```python
from build123d import *

# Parameters (mm, degrees)
SKETCH_1_R          = 8
SKETCH_1_R_2        = 6
EXTRUDE_1_DEPTH     = 2
SKETCH_1_3_R        = 6
SKETCH_1_3_R_2      = 1.65
EXTRUDE_2_DEPTH     = 35
SKETCH_2_R          = 1
CUT_EXTRUDE_1_DEPTH = 2
CUT_EXTRUDE_START   = 35
SKETCH_1_4_R        = 1.65
CUT_EXTRUDE_2_DEPTH = 13
CHAMFER_1_SIZE      = 0.2
CHAMFER_2_SIZE      = 0.3


with BuildPart() as part:
    # 스케치1 → 보스-돌출1 (new body)
    with BuildSketch(Plane(origin=(0, 0, 0), x_dir=(1, 0, 0), z_dir=(0, 1, 0))):
        with Locations(Location((0, 0, 0), (0, 0, 270))):
            Circle(SKETCH_1_R)
        with Locations(Location((0, 0, 0), (0, 0, 270))):
            Circle(SKETCH_1_R_2, mode=Mode.SUBTRACT)
    extrude(amount=EXTRUDE_1_DEPTH)

    # 스케치1<3> → 보스-돌출2 (add)
    # profile 1 of 2: a face of its own
    with BuildSketch(Plane(origin=(0, 0, 0), x_dir=(1, 0, 0), z_dir=(0, 1, 0))):
        with Locations(Location((0, 0, 0), (0, 0, 270))):
            Circle(SKETCH_1_3_R)
        Circle(SKETCH_1_3_R_2, mode=Mode.SUBTRACT)
    # profile 2 of 2: a face of its own
    with BuildSketch(Plane(origin=(0, 0, 0), x_dir=(1, 0, 0), z_dir=(0, 1, 0))):
        Circle(SKETCH_1_3_R_2)
    extrude(amount=EXTRUDE_2_DEPTH)

    # 스케치2 → 컷-돌출1 (cut)
    with BuildSketch(Plane.XZ):
        with Locations((0, 3)):
            Circle(SKETCH_2_R)
        with BuildLine():
            ThreePointArc((1, 3), (0, 2), (-1, 3))
            Line((-1, 3), (-1, -3))
            ThreePointArc((-1, -3), (0, -2), (1, -3))
            Line((1, -3), (1, 3))
        make_face()
        with Locations((0, -3)):
            Circle(SKETCH_2_R)
    extrude(amount=-CUT_EXTRUDE_1_DEPTH, mode=Mode.SUBTRACT)

    # 스케치1<4> → 컷-돌출2 (cut)
    with BuildSketch(Plane(origin=(0, 0, 0), x_dir=(1, 0, 0), z_dir=(0, 1, 0)).offset(CUT_EXTRUDE_START)):
        with Locations(Location((0, 0, 0), (0, 0, 270))):
            Circle(SKETCH_1_4_R)
    extrude(amount=-CUT_EXTRUDE_2_DEPTH, mode=Mode.SUBTRACT)

    # 모따기1
    chamfer_1_edges = [part.edges().sort_by_distance(p)[0] for p in [
        (0, 2, -8),
        (0, 35, -1.65),
        (0, 0, -8),
    ]]
    chamfer(chamfer_1_edges, length=CHAMFER_1_SIZE)

    # 모따기2
    chamfer_2_edges = [part.edges().sort_by_distance(p)[0] for p in [
        (0, 35, -6),
    ]]
    chamfer(chamfer_2_edges, length=CHAMFER_2_SIZE)

    # 스케치3 → 컷-회전1 (revolve, cut)
    with BuildSketch(Plane.XY, mode=Mode.PRIVATE) as cut_revolve_1_sk:
        Polygon((-1.65, 22), (0, 21.316547622), (0, 22), align=None)
    revolve(cut_revolve_1_sk.sketch.rotate(Axis((0, -0.686408766, 0), (0, 1, 0)), 90), axis=Axis((0, -0.686408766, 0), (0, 1, 0)), mode=Mode.SUBTRACT)


solid = part.part
```
Verification items for the finished model (mm, model axes). A direction names the side the tool comes from. Coordinates: 2 decimals unless noted, no trailing zeros. Order: outer loops, then holes, each group sorted by start corner. A loop starts at its lowest first (then second) coordinate and runs counter-clockwise, first axis right, second up. Notation, with made-up numbers: (33, -14.75) - (51, -14.75) arc R11 ccw to (51, 6.25) - close; hole circle Ø5 at (76, -22.75). An arc over 180 degrees is marked (long way). Return JSON: item names as keys, results as strings.
(1) Access from +Z, -Z, +X, -X, +Y, -Y to the whole of each face (thin tool, end or side, straight path). Record for faces 1 (the flat face through (-5, 2, 4)), 2 (the flat face through (-2, 35, 0)), 3 (the cylindrical face through (0, 1, 4)).
Filled sheet:
{"face 1": "+Y", "face 2": "+Z, -Z, +X, -X, +Y", "face 3": "-Y"}
(2) Thickness scan on line 1 along X through (y, z) = (32.25, 0); line 2 along Y through (x, z) = (6.25, -0.5); line 3 along X through (y, z) = (23.5, 1.5). Record the ranges inside material, lowest first.
Filled sheet:
{"line 1": "x = -6 to -1.65, 1.65 to 6", "line 2": "y = 0 to 2", "line 3": "x = -5.81 to -0.69, 0.69 to 5.81"}
(3) Mould release check, pull along Z, two halves, no side actions. Record for faces 4 (the cylindrical face through (0, 1, -4)), 5 (the flat face through (-2, 0, 0)), 6 (the cylindrical face through (1.802, 18.121, 5.723)): pulls with the +Z half, pulls with the -Z half, needs draft (parallel to the pull), parting line crosses it, or undercut.
Filled sheet:
{"face 4": "undercut", "face 5": "needs draft", "face 6": "parting line crosses it"}
(4) Go/stop test with flat-tipped pins: pin 1 (5 mm diameter, centred on y = 10, z = -2, fed in from -X); pin 2 (1.5 mm diameter, centred on x = -0.5, y = 27, fed in from +Z); pin 3 (1.5 mm diameter, centred on x = 4.5, y = 26.5, fed in from -Z). Record where each tip stops, or that it passes through.
Filled sheet:
{"pin 1": "stops at x = -6", "pin 2": "stops at z = 6", "pin 3": "stops at z = -4.68"}
(5) Section check A-A, the plane y = 18. Record the cut outline in (x, z), and give its area (3 significant figures).
Filled sheet:
{"outline": "circle Ø12 at (0, 0)", "area": "113 mm^2"}
